```python
from build123d import *

# Parameters (mm, degrees)
ESTRUSIONE_ESTRUSIONE1_DEPTH                         = 3
ESTRUSIONE_ESTRUSIONE1_DEPTH_BACK                    = 17
TAGLIO_ESTRUSIONE1_DEPTH                             = 3
FORO_LAMATO_PER_VITE_M6_A_TESTA_CILINDRI_D           = 6.4
FORO_LAMATO_PER_VITE_M6_A_TESTA_CILINDRI_CBORE_D     = 11
FORO_LAMATO_PER_VITE_M6_A_TESTA_CILINDRI_CBORE_DEPTH = 6.4
RIPETIZIONECIRCOLARE1_COUNT                          = 2
FORO_PER_VITE_M6_1_D                                 = 6.6


with BuildPart() as part:
    # Schizzo2 → Estrusione-Estrusione1 (new body, two sides)
    with BuildSketch(Plane.XY) as estrusione_estrusione1_sk:
        with BuildLine():
            Line((-222.25, -85), (335.6, -85))
            ThreePointArc((335.6, -85), (342.671067812, -82.071067812), (345.6, -75))
            Line((345.6, -75), (345.6, 75))
            ThreePointArc((345.6, 75), (342.671067812, 82.071067812), (335.6, 85))
            Line((335.6, 85), (-222.25, 85))
            ThreePointArc((-222.25, 85), (-229.321067812, 82.071067812), (-232.25, 75))
            Line((-232.25, 75), (-232.25, -75))
            ThreePointArc((-232.25, -75), (-229.321067812, -82.071067812), (-222.25, -85))
        make_face()
    extrude(amount=ESTRUSIONE_ESTRUSIONE1_DEPTH)
    extrude(estrusione_estrusione1_sk.sketch, amount=-ESTRUSIONE_ESTRUSIONE1_DEPTH_BACK)

    # Schizzo3 → Taglio-Estrusione1 (cut)
    with BuildSketch(Plane.XY.offset(3)):
        with BuildLine():
            Line((-127.822135955, 62), (-232.25, 62))
            Line((-232.25, 62), (-232.25, -62))
            Line((-232.25, -62), (-127.822135955, -62))
            ThreePointArc((-127.822135955, -62), (-127.005639374, -62.174258142), (-126.33142397, -62.666666667))
            ThreePointArc((-126.33142397, -62.666666667), (-120.521572875, -62.828427125), (-120.683333333, -57.01857603))
            ThreePointArc((-120.683333333, -57.01857603), (-121.175741858, -56.344360626), (-121.35, -55.527864045))
            Line((-121.35, -55.527864045), (-121.35, 55.527864045))
            ThreePointArc((-121.35, 55.527864045), (-121.175741858, 56.344360626), (-120.683333333, 57.01857603))
            ThreePointArc((-120.683333333, 57.01857603), (-120.521572875, 62.828427125), (-126.33142397, 62.666666667))
            ThreePointArc((-126.33142397, 62.666666667), (-127.005639374, 62.174258142), (-127.822135955, 62))
        make_face()
    taglio_estrusione1 = extrude(amount=-TAGLIO_ESTRUSIONE1_DEPTH, mode=Mode.SUBTRACT)

    # Foro lamato per Vite M6 a testa cilindri (through all)
    with Locations(Plane(origin=(0, 0, -17), x_dir=(-1, 0, 0), z_dir=(0, 0, -1))):
        with Locations((136.35, -42.588457268), (136.35, 32.411542732), (218.35, 32.411542732)):
            foro_lamato_per_vite_m6_a_testa_cilindri = CounterBoreHole(FORO_LAMATO_PER_VITE_M6_A_TESTA_CILINDRI_D / 2, FORO_LAMATO_PER_VITE_M6_A_TESTA_CILINDRI_CBORE_D / 2, FORO_LAMATO_PER_VITE_M6_A_TESTA_CILINDRI_CBORE_DEPTH)

    # RipetizioneCircolare1: Taglio-Estrusione1, Foro lamato per Vite M6 a testa cilindri ×2 about axis
    ripetizionecircolare1_axis = Axis((56.675, 0, 0), (0, 0, 1))
    add([taglio_estrusione1.rotate(ripetizionecircolare1_axis, i * 360 / RIPETIZIONECIRCOLARE1_COUNT) for i in range(1, RIPETIZIONECIRCOLARE1_COUNT)], mode=Mode.SUBTRACT)
    add([foro_lamato_per_vite_m6_a_testa_cilindri.rotate(ripetizionecircolare1_axis, i * 360 / RIPETIZIONECIRCOLARE1_COUNT) for i in range(1, RIPETIZIONECIRCOLARE1_COUNT)], mode=Mode.SUBTRACT)

    # Foro per Vite M6-1 (through all)
    with Locations(Plane.XY.offset(3)):
        with Locations((-93.325, 25), (206.675, -25), (-93.325, -25), (206.675, 25), (56.675, 25), (56.675, -25), (-43.325, 25), (-43.325, -25), (6.675, -25), (6.675, 25), (106.675, -25), (106.675, 25), (156.675, 25), (156.675, -25)):
            Hole(FORO_PER_VITE_M6_1_D / 2)


solid = part.part
```
CAD build for the part. Positions are in the model's coordinates, mm. A direction names the side the tool comes from. Round coordinates to 2 decimals unless told otherwise and drop trailing zeros. Loops run counter-clockwise (first coordinate to the right, second up) from the corner with the lowest first, then second, coordinate; pieces in that order, holes last. Notation, with made-up numbers: (54, -3.75) - (99, -3.75) arc R30 ccw to (99, 35.25) - close; hole circle Ø10 at (-15, 45.25). An arc over 180 degrees is marked (long way). Return JSON: item names as keys, results as strings. Group by question number.
Q1. Band-saw the part on A-A on x = 269. Give the cut face in (y, z).
Q2. Drill centre lines: line 1 along X through (y, z) = (33, -14.5); line 2 along X through (y, z) = (42.5, -8); line 3 along X through (y, z) = (-34.5, -2.5). Where is each one in solid material? Low to high. Write a range as [from, to].
Q3. Flat gauge pins, fed straight in: pin 1 Ø2.5 at (y, z) = (-3.5, 1.5) entering from -X; pin 2 Ø7.5 at (x, y) = (249.7, 42.59) entering from -Z; pin 3 Ø12 at (x, y) = (242, 29) entering from +Z. Where does each tip first touch, or does it go through?
Q4. Tool access for faces 5 (the face through (61, 85, -7)), 6 (the face through (254.781, -30.305, -13.845)): list every direction of +Z, -Z, +X, -X, +Y, -Y with a clear straight run to the whole face (end or side of a thin tool).
Q5. Two-plate mould, pull along X, no slides. Class faces 1 (the face through (-229.4, -81.99, -6.86)), 2 (the face through (-139, -45, -10.6)), 3 (the face through (342.75, 81.99, -6.86)), 4 (the face through (252.1, -30, -10.6)): +X half, -X half, draft (parallel to the pull), parting line (faces both ways), or undercut.
Q6. Band-saw the part on B-B on y = 4.5. Give the cut face in (x, z), plus the area to 3 significant figures.
Solutions:
{
 "1": {"outline": "(-85, -17) - (85, -17) - (85, 3) - (62, 3) - (62, 0) - (-62, 0) - (-62, 3) - (-85, 3) - close"},
 "2": {"line 1": "x = [-232.25, -223.82], [-212.88, -141.82], [-130.88, 345.6]", "line 2": "x = [-232.25, 246.5], [252.9, 345.6]", "line 3": "x = [-232.25, 247.28], [252.12, 329.28], [334.12, 345.6]"},
 "3": {"pin 1": "stops at x = -121.35", "pin 2": "stops at z = -10.6", "pin 3": "stops at z = 0"},
 "4": {"face 5": "+Z, -Z, +X, -X, +Y", "face 6": "-Z"},
 "5": {"face 1": "-X half", "face 2": "undercut", "face 3": "+X half", "face 4": "undercut"},
 "6": {"outline": "(-232.25, -17) - (345.6, -17) - (345.6, 0) - (234.7, 0) - (234.7, 3) - (-121.35, 3) - (-121.35, 0) - (-232.25, 0) - close", "area": "10,900 mm^2"}
}
